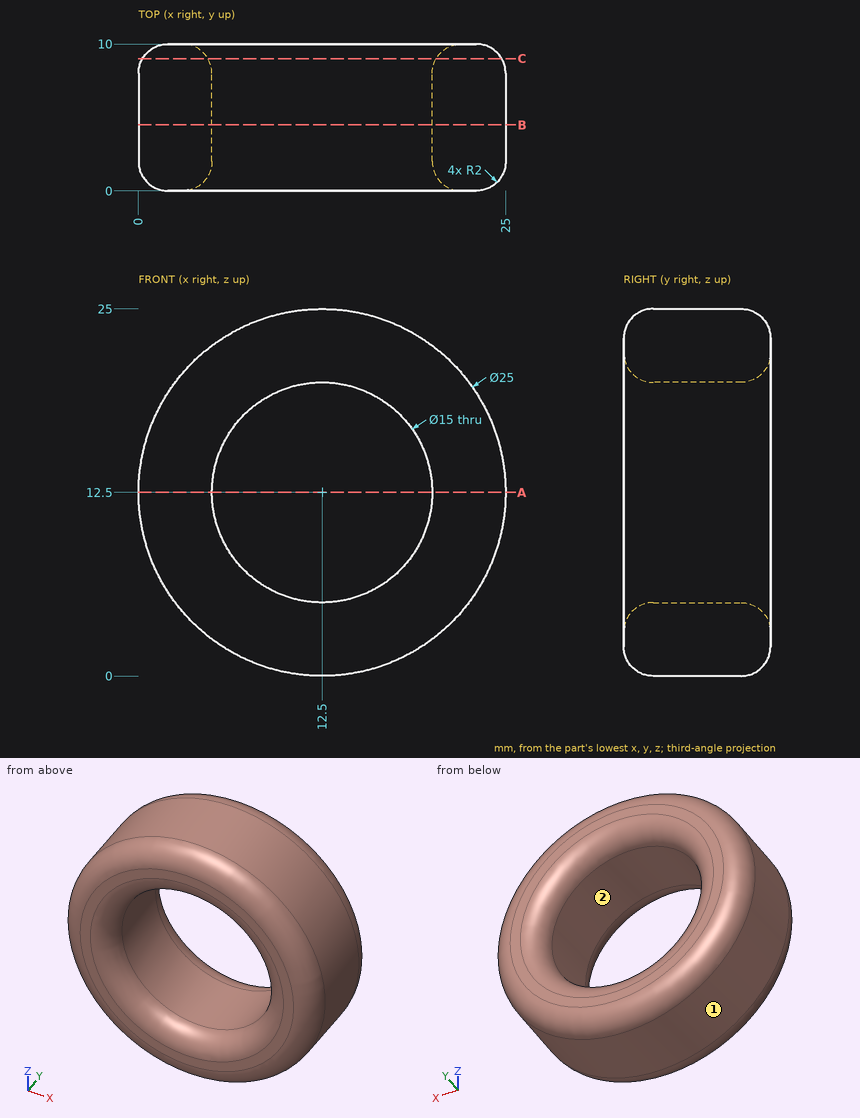
Verification items for this drawing (mm, ordinates from the low corner). Round coordinates to 2 decimals unless told otherwise and drop trailing zeros. Loops run counter-clockwise (first coordinate to the right, second up) from the corner with the lowest first, then second, coordinate; pieces in that order, holes last. Notation, with made-up numbers: (34.5, -31.5) - (75.5, -31.5) arc R12 ccw to (75.5, -14.5) - close; hole circle Ø4 at (72.5, -6). An arc over 180 degrees is marked (long way). Answer as CSV lines item,"result". Start each with the question number.
Item 1: Depth check by flat-ended pin: P1, Ø4, axis at x = 10.5, y = 1, coming from the -Z side; P2, Ø3, axis at y = 5, z = 17, coming from the -X side; P3, Ø2, axis at x = 3, y = 2.5, coming from the +Z side. Enter the tip coordinate at first touch or a pass-through.
Item 2: Section check C-C (y = 9). Record the boundary of the cut face in (x, z), and give its area (3 significant figures).
Item 3: Section check B-B (y = 4.5). Record the boundary of the cut face in (x, z), and give its area (3 significant figures).
Item 4: Scan lines: line 1 (X direction, y = 6.65, z = 12.5); line 2 (Z direction, x = 7.5, y = 7.25); line 3 (Z direction, x = 2.5, y = 5). Record each from-to range of solid material in increasing order. Write a range as [from, to].
Item 5: Section check A-A (z = 12.5). Record the boundary of the cut face in (x, y), and give its area (3 significant figures).
Item 6: Release check for a two-part mould opening along Z. For the marked faces 1 and 2 record: +Z half, -Z half, draft (parallel to the pull), parting line (faces both ways), or undercut.
Report:
1,P1,"stops at z = 0"
1,P2,"stops at x = 0.37"
1,P3,"stops at z = 21.67"
2,outline,"circle Ø24.46 at (12.5, 12.5); hole circle Ø15.54 at (12.5, 12.5)"
2,area,"280 mm2"
3,outline,"circle Ø25 at (12.5, 12.5); hole circle Ø15 at (12.5, 12.5)"
3,area,"314 mm2"
4,line 1,"x = [0, 5], [20, 25]"
4,line 2,"z = [1.04, 6.91], [18.09, 23.96]"
4,line 3,"z = [5, 20]"
5,outline,"(0, 2) arc R2 ccw to (2, 0) - (3, 0) arc R2 ccw to (5, 2) - (5, 8) arc R2 ccw to (3, 10) - (2, 10) arc R2 ccw to (0, 8) - close; (20, 2) arc R2 ccw to (22, 0) - (23, 0) arc R2 ccw to (25, 2) - (25, 8) arc R2 ccw to (23, 10) - (22, 10) arc R2 ccw to (20, 8) - close"
5,area,"93.1 mm2"
6,face 1,"parting line"
6,face 2,"undercut"
